from build123d import *

# Parameters (mm, degrees)
BOSS_EXTRUDE1_DEPTH = 500
CHAMFER2_SIZE       = 0.5
CHAMFER2_SIZE2      = 0.353553391
CHAMFER1_SIZE       = 0.5


with BuildPart() as part:
    # Sketch1 → Boss-Extrude1 (new body)
    with BuildSketch(Plane.XY):
        with BuildLine():
            Line((5.5, 6.829360749), (2.570639251, 3.9))
            Line((2.570639251, 3.9), (0, 3.9))
            Line((0, 3.9), (0, 2.1))
            ThreePointArc((0, 2.1), (0.803635208, 1.940147018), (1.48492424, 1.48492424))
            Line((1.48492424, 1.48492424), (10, 10))
            Line((10, 10), (4.5, 10))
            Line((4.5, 10), (2.62, 8.12))
            Line((2.62, 8.12), (5.5, 8.12))
            Line((5.5, 8.12), (5.5, 6.829360749))
        make_face()
    extrude(amount=BOSS_EXTRUDE1_DEPTH)

    # Chamfer2
    chamfer2_edges = [part.edges().sort_by_distance(p)[0] for p in [
        (2.62, 8.12, 250),
    ]]
    chamfer2_side = [part.faces().sort_by_distance(p)[0] for p in [
        (3.56, 9.06, 250),
    ]]
    chamfer(chamfer2_edges, length=CHAMFER2_SIZE, length2=CHAMFER2_SIZE2, reference=chamfer2_side[0])

    # Mirror1: part across plane


with BuildPart() as part_1:
    add(part.part)
    add(part.part.mirror(Plane(origin=(10, 10, 500), x_dir=(0, 0, 1), z_dir=(-0.707106781186544, 0.7071067811865511, 0))))

    # Chamfer1
    chamfer1_edges = [part_1.edges().sort_by_distance(p)[0] for p in [
        (10, 10, 250),
    ]]
    chamfer(chamfer1_edges, length=CHAMFER1_SIZE)

    # Mirror4: part across plane


with BuildPart() as part_2:
    add(part_1.part)
    add(part_1.part.mirror(Plane(origin=(0, 3.9, 500), x_dir=(0, 0, 1), z_dir=(1, 0, 0))))

    # Mirror5: part across plane


with BuildPart() as part_3:
    add(part_2.part)
    add(part_2.part.mirror(Plane(origin=(-3.9, 0, 500), x_dir=(0, 0, 1), z_dir=(0, 1, 0))))


solid = part_3.part
Part model, mm, in its own coordinate system. Give positions to 0.01 mm unless a question says otherwise; leave off trailing zeros. One line per question, with ' | ' between items.
1. Pull direction Z, two halves, no side cores. Call faces 1 (the face through (-2.4, 0.1, 0)), 2 (the face through (-2.4, 0.1, 500)): +Z half, -Z half, draft (parallel to the pull), parting line (faces both ways), or undercut.
Filled in:
face 1: -Z half | face 2: +Z half
2. Drill centre lines: probe 1 along X at (y, z) = (7, 173); probe 2 along X at (y, z) = (-8.5, 325); probe 3 along X at (y, z) = (4.5, 99). Where is each one in solid material? Low to high.
Filled in:
probe 1: -10 to -5.5, 5.5 to 10 | probe 2: -10 to -3, 3 to 10 | probe 3: -10 to -8.12, -5.83 to -3.17, 3.17 to 5.83, 8.12 to 10
3. Drop flat-ended pins along their axis: P1, Ø10, axis at x = 4, y = 7, coming from the -Z side; P2, Ø5, axis at y = 1.5, z = 365.5, coming from the +X side; P3, Ø2.5, axis at x = 1, z = 161.5, coming from the -Y side; P4, Ø5.5, axis at y = 0, z = 240.5, coming from the -X side. Give the stop position or say it passes through.
Filled in:
P1: z = 0 | P2: x = 9.5 | P3: y = -3.9 | P4: x = -4.08
